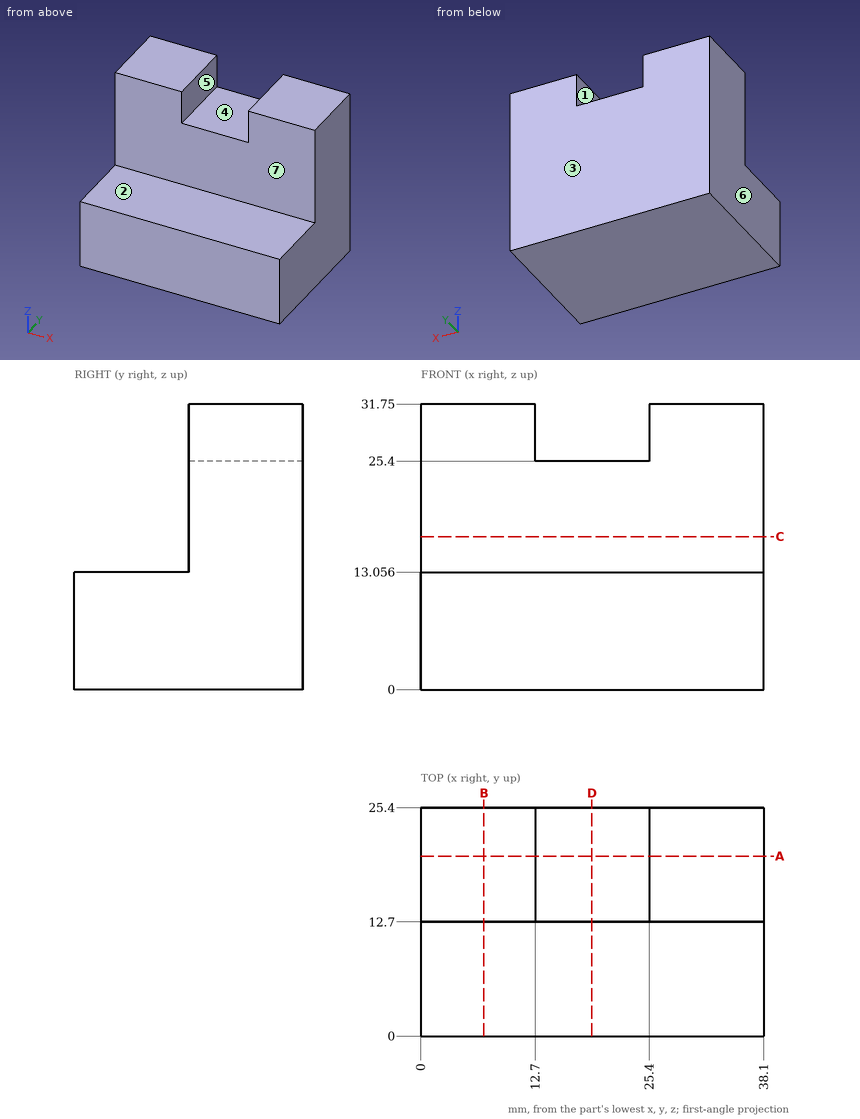
Here's the drawing with two shaded views (mm, measured from the low corner). I have some questions. A direction names the side the tool comes from. Coordinates: 2 decimals unless noted, no trailing zeros. Order: outer loops, then holes, each group sorted by start corner. A loop starts at its lowest first (then second) coordinate and runs counter-clockwise, first axis right, second up.
Item 1: Thinking about a two-plate mould opening in X: for the marked faces 4, 5, 6 and 7, which applies, pulls with the +X half, pulls with the -X half, needs draft (parallel to the pull), parting line crosses it, or undercut?
Response values:
face 4: undercut
face 5: undercut
face 6: pulls with the -X half
face 7: needs draft
Item 2: Which directions (+Z, -Z, +X, -X, +Y, -Y) give clear straight access to the entire face, cutting with the end or side of a thin tool? Please do the marked faces 1, 2 and 3.
Response values:
face 1: +Z, +Y, -Y
face 2: +Z, +X, -X, -Y
face 3: +Z, -Z, +X, -X, +Y
Item 3: If we section it at C-C, the plane z = 17: List the corners of the cut face in (x, y) for me, then the cut area to 3 significant figures.
Response values:
outline: (0, 12.7) - (38.1, 12.7) - (38.1, 25.4) - (0, 25.4) - close
area: 484 mm2
Item 4: I'm going to push flat-ended pins straight in: pin 1 Ø15 at (x, z) = (12, 23.5) entering from -Y; pin 2 Ø1 at (x, y) = (16.5, 21) entering from +Z; pin 3 Ø10 at (x, y) = (11.5, 4.5) entering from +Z. Where does each tip first touch, or does it pass through?
Response values:
pin 1: stops at y = 12.7
pin 2: stops at z = 25.4
pin 3: stops at z = 13.06
Item 5: I need wall thicknesses on probe 1 along Y at (x, z) = (33, 17); probe 2 along Z at (x, y) = (16.5, 6); probe 3 along Z at (x, y) = (21, 18.25). Which ranges of each line are inside material? Lowest first, please.
Response values:
probe 1: y = 12.7 to 25.4
probe 2: z = 0 to 13.06
probe 3: z = 0 to 25.4
Item 6: If we section it at B-B, the plane x = 7: List the corners of the cut face in (y, z) for me, then the cut area to 3 significant figures.
Response values:
outline: (0, 0) - (25.4, 0) - (25.4, 31.75) - (12.7, 31.75) - (12.7, 13.06) - (0, 13.06) - close
area: 569 mm2
Item 7: If we section it at A-A, the plane y = 20: List the corners of the cut face in (x, z) for me.
Response values:
outline: (0, 0) - (38.1, 0) - (38.1, 31.75) - (25.4, 31.75) - (25.4, 25.4) - (12.7, 25.4) - (12.7, 31.75) - (0, 31.75) - close
Item 8: If we section it at D-D, the plane x = 19: List the corners of the cut face in (y, z) for me.
Response values:
outline: (0, 0) - (25.4, 0) - (25.4, 25.4) - (12.7, 25.4) - (12.7, 13.06) - (0, 13.06) - close
